Build history of the part. All positions in model axes, mm. Coordinates: 2 decimals unless noted, no trailing zeros. Order: outer loops, then holes, each group sorted by start corner. A loop starts at its lowest first (then second) coordinate and runs counter-clockwise, first axis right, second up. Notation, with made-up numbers: (12.5, 31) - (50.5, 31) arc R12 ccw to (50.5, 44) - close; hole circle Ø10 at (13, -27.5). An arc over 180 degrees is marked (long way). Return JSON: item names as keys, results as strings.
from build123d import *

# Parameters (mm, degrees)
SKETCH1_W           = 38.1
SKETCH1_H           = 50.8
SKETCH1_R           = 1.5
BOSS_EXTRUDE1_DEPTH = 1.5
SKETCH2_R           = 0.889
CUT_EXTRUDE1_DEPTH  = 32.785413321
SKETCH3_W           = 1.016
SKETCH3_H           = 1.016
BOSS_EXTRUDE2_DEPTH = 5.08


with BuildPart() as part:
    # Sketch1 → Boss-Extrude1 (new body)
    with BuildSketch(Plane.XY):
        Rectangle(SKETCH1_W, SKETCH1_H)
        with Locations((-17.018, -23.368)):
            Circle(SKETCH1_R, mode=Mode.SUBTRACT)
        with Locations((-15.875, 22.225)):
            Circle(SKETCH1_R, mode=Mode.SUBTRACT)
        with Locations(Location((17.018, -23.368, 0), (0, 0, 180))):
            Circle(SKETCH1_R, mode=Mode.SUBTRACT)
        with Locations(Location((15.875, 22.225, 0), (0, 0, 180))):
            Circle(SKETCH1_R, mode=Mode.SUBTRACT)
    extrude(amount=BOSS_EXTRUDE1_DEPTH)

    # Sketch2 → Cut-Extrude1 (cut, through all)
    with BuildSketch(Plane.XY.offset(1.5)):
        with Locations((17.272, -11.684)):
            Circle(SKETCH2_R)
        with Locations((17.272, -5.08)):
            Circle(SKETCH2_R)
    extrude(amount=-CUT_EXTRUDE1_DEPTH, mode=Mode.SUBTRACT)

    # Sketch3 → Boss-Extrude2 (add)
    with BuildSketch(Plane.XY.offset(1.5)):
        with Locations((-13.97, -23.876)):
            Rectangle(SKETCH3_W, SKETCH3_H)
        with Locations((-13.97, -21.336)):
            Rectangle(SKETCH3_W, SKETCH3_H)
        with Locations((-13.97, -18.796)):
            Rectangle(SKETCH3_W, SKETCH3_H)
        with Locations((-13.97, -16.256)):
            Rectangle(SKETCH3_W, SKETCH3_H)
        with Locations((-11.176, -23.876)):
            Rectangle(SKETCH3_W, SKETCH3_H)
        with Locations((-11.176, -21.336)):
            Rectangle(SKETCH3_W, SKETCH3_H)
        with Locations((-11.176, -18.796)):
            Rectangle(SKETCH3_W, SKETCH3_H)
        with Locations((-11.176, -16.256)):
            Rectangle(SKETCH3_W, SKETCH3_H)
        with Locations((-8.382, -23.876)):
            Rectangle(SKETCH3_W, SKETCH3_H)
        with Locations((-8.382, -21.336)):
            Rectangle(SKETCH3_W, SKETCH3_H)
        with Locations((-8.382, -18.796)):
            Rectangle(SKETCH3_W, SKETCH3_H)
        with Locations((-8.382, -16.256)):
            Rectangle(SKETCH3_W, SKETCH3_H)
        with Locations((-2.794, -23.876)):
            Rectangle(SKETCH3_W, SKETCH3_H)
        with Locations((-2.794, -21.336)):
            Rectangle(SKETCH3_W, SKETCH3_H)
        with Locations((-2.794, -18.796)):
            Rectangle(SKETCH3_W, SKETCH3_H)
        with Locations((-2.794, -16.256)):
            Rectangle(SKETCH3_W, SKETCH3_H)
        with Locations((0, -23.876)):
            Rectangle(SKETCH3_W, SKETCH3_H)
        with Locations((0, -21.336)):
            Rectangle(SKETCH3_W, SKETCH3_H)
        with Locations((0, -18.796)):
            Rectangle(SKETCH3_W, SKETCH3_H)
        with Locations((0, -16.256)):
            Rectangle(SKETCH3_W, SKETCH3_H)
        with Locations((2.794, -23.876)):
            Rectangle(SKETCH3_W, SKETCH3_H)
        with Locations((2.794, -21.336)):
            Rectangle(SKETCH3_W, SKETCH3_H)
        with Locations((2.794, -18.796)):
            Rectangle(SKETCH3_W, SKETCH3_H)
        with Locations((2.794, -16.256)):
            Rectangle(SKETCH3_W, SKETCH3_H)
        with Locations((8.382, -23.876)):
            Rectangle(SKETCH3_W, SKETCH3_H)
        with Locations((8.382, -21.336)):
            Rectangle(SKETCH3_W, SKETCH3_H)
        with Locations((8.382, -18.796)):
            Rectangle(SKETCH3_W, SKETCH3_H)
        with Locations((8.382, -16.256)):
            Rectangle(SKETCH3_W, SKETCH3_H)
        with Locations((11.176, -23.876)):
            Rectangle(SKETCH3_W, SKETCH3_H)
        with Locations((11.176, -21.336)):
            Rectangle(SKETCH3_W, SKETCH3_H)
        with Locations((11.176, -18.796)):
            Rectangle(SKETCH3_W, SKETCH3_H)
        with Locations((11.176, -16.256)):
            Rectangle(SKETCH3_W, SKETCH3_H)
        with Locations((13.97, -23.876)):
            Rectangle(SKETCH3_W, SKETCH3_H)
        with Locations((13.97, -21.336)):
            Rectangle(SKETCH3_W, SKETCH3_H)
        with Locations((13.97, -18.796)):
            Rectangle(SKETCH3_W, SKETCH3_H)
        with Locations((13.97, -16.256)):
            Rectangle(SKETCH3_W, SKETCH3_H)
    extrude(amount=BOSS_EXTRUDE2_DEPTH)


solid = part.part
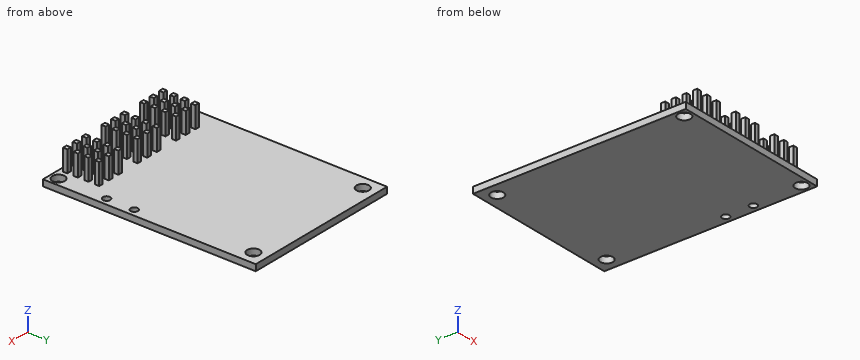
1. Drop flat-ended pins along their axis: pin 1 (2 mm diameter, centred on y = -16.5, z = 3.5, fed in from +X); pin 2 (3 mm diameter, centred on x = 14, z = 4, fed in from +Y); pin 3 (1.5 mm diameter, centred on x = 6, y = -5, fed in from +Z). Give the stop position or say it passes through.
Check values:
{"pin 1": "x = 14.48", "pin 2": "y = -15.75", "pin 3": "z = 1.5"}
2. Cut at D-D on x = 12.5. Give the cut face in (y, z).
Check values:
{"outline": "(-25.4, 0) - (25.4, 0) - (25.4, 1.5) - (-25.4, 1.5) - close"}
3. Cut at B-B on z = 2.5. State how many separate pieces and enclosed holes the cut face has, plus the area to 3 significant figures.
Check values:
{"separate pieces": "36", "enclosed holes": "0", "area": "37.2 mm²"}
4. Cut at A-A on y = -5.08. Give the cut face in (x, z), plus the area to 3 significant figures.
Check values:
{"outline": "(-19.05, 0) - (16.38, 0) - (16.38, 1.5) - (-19.05, 1.5) - close; (18.16, 0) - (19.05, 0) - (19.05, 1.5) - (18.16, 1.5) - close", "area": "54.5 mm²"}
5. Probe L1, parallel to Y at x = 13.5, z = 3.75; L2, parallel to Z at x = -9, y = 6. List the from-to ranges inside material, lowest first.
Check values:
{"L1": "-24.38 to -23.37, -21.84 to -20.83, -19.3 to -18.29, -16.76 to -15.75", "L2": "0 to 1.5"}
6. Cut at C-C on y = 13.5. Give the cut face in (x, z), plus the area to 4 significant figures.
Check values:
{"outline": "(-19.05, 0) - (19.05, 0) - (19.05, 1.5) - (-19.05, 1.5) - close", "area": "57.15 mm²"}
